Geometry check sheet. Reference: the model listing, model coordinates, mm. A direction names the side the tool comes from. Round coordinates to 2 decimals unless told otherwise and drop trailing zeros. Order: outer loops, then holes, each group sorted by start corner. A loop starts at its lowest first (then second) coordinate and runs counter-clockwise, first axis right, second up. Notation, with made-up numbers: M 75,-11.75 L 94,-11.75 A19 ccw 94,0.25 Z; hole C 60,-4.75 d1. An arc over 180 degrees is marked long. Answer as a JSON object with one key per item and string values. Group by question number.
Autodesk Fusion 360 part; units mm, degrees
sketch "Skizze1" plane through (0, 0, 0) normal (0, 0, 1) x (1, 0, 0)
  line L0 (0, 0) -> (17, 0)
  line L1 (17, 0) -> (17, 27)
  line L2 (17, 27) -> (0, 27)
  line L3 (0, 27) -> (0, 0)
  line L4 (14, 27) -> (12.5, 25.5)
  line L5 (12.5, 25.5) -> (4.5, 25.5)
  line L6 (4.5, 25.5) -> (3, 27)
  line L7 (4.5, 27) -> (12.5, 27)
  line L8 (12.5, 27) -> (12.5, 21)
  line L9 (12.5, 21) -> (4.5, 21)
  line L10 (4.5, 21) -> (4.5, 27)
  circle A0 centre (2, 25) radius 0.5
  circle A1 centre (15, 25) radius 0.5
  circle A2 centre (2, 2) radius 0.5
  circle A3 centre (15, 2) radius 0.5
  circle A4 centre (7.23, 2) radius 0.5
  circle A5 centre (9.77, 2) radius 0.5
  line L11 (8.5, 0) -> (8.5, 3.6203)
  circle A6 centre (1.5, 5.5) radius 0.5
  circle A7 centre (1.5, 8.04) radius 0.5
  circle A8 centre (1.5, 15.66) radius 0.5
  circle A9 centre (1.5, 18.2) radius 0.5
  dimension "d1" = 17
  dimension "d2" = 27
  dimension "d3" = 3
  dimension "d4" = 3
  dimension "d5" = 45
  dimension "d6" = 45
  dimension "d7" = 1.5
  dimension "d8" = 8
  dimension "d9" = 6
  dimension "d10" = 4.5
  dimension "d17" = 1
  dimension "d18" = 2
  dimension "d19" = 2
  dimension "d22" = 13
  dimension "d23" = -23
  dimension "d24" = 1
  dimension "d25" = 2
  dimension "d28" = 2.54
  dimension "d29" = 0
  dimension "d30" = 1
  dimension "d31" = 5.5
  dimension "d32" = 1.5
  dimension "d35" = 0
  dimension "d36" = 2.54
  dimension "d39" = 0
  dimension "d40" = 10.16
extrude "Extrusion2" add sketch "Skizze1" along normal blind 4 contours L2 L5 L7 L8 L10 | L5 L8 L9 L10
extrude "Extrusion3" cut sketch "Skizze1" along normal blind 1.6 contours L2 L5 L7 L8 L10
extrude "Extrusion4" add sketch "Skizze1" along normal blind 1.6 contours L0 L1 L2 L3 L4 L6 L8 L9 L10
sketch "Skizze2" plane through (0, 0, 1.6) normal (0, 0, 1) x (-1, 0, 0)
  circle A0 centre (-1.5, -15.66) radius 0.5
  circle A1 centre (-2, -2) radius 0.5
  circle A2 centre (-1.5, -8.04) radius 0.5
  circle A3 centre (-15, -25) radius 0.5
  circle A4 centre (-1.5, -18.2) radius 0.5
  circle A5 centre (-7.23, -2) radius 0.5
  circle A6 centre (-1.5, -5.5) radius 0.5
  circle A7 centre (-15, -2) radius 0.5
  circle A8 centre (-9.77, -2) radius 0.5
  circle A9 centre (-2, -25) radius 0.5
  line L0 (-4.5, -21) -> (-4.5, -25.5)
  line L1 (-4.5, -25.5) -> (-3, -27)
  line L2 (-3, -27) -> (0, -27)
  line L3 (0, -27) -> (0, 0)
  line L4 (0, 0) -> (-17, 0)
  line L5 (-17, 0) -> (-17, -27)
  line L6 (-17, -27) -> (-14, -27)
  line L7 (-14, -27) -> (-12.5, -25.5)
  line L8 (-12.5, -25.5) -> (-12.5, -21)
  line L9 (-12.5, -21) -> (-4.5, -21)
  line L10 (-4.75, -3.5) -> (-12.25, -3.5)
  line L11 (-12.25, -3.5) -> (-12.25, 7.5)
  line L12 (-12.25, 7.5) -> (-4.75, 7.5)
  line L13 (-4.75, 7.5) -> (-4.75, -3.5)
  line L14 (-4.75, 0) -> (-12.25, 0)
  line L15 (0, 0) -> (-17, 0)
  dimension "d43" = 7.5
  dimension "d44" = 11
  dimension "d45" = 3.5
extrude "Extrusion5" [suppressed]
1) Sectioned sample at D-D (x = 9.77). Record the boundary of the cut face in (y, z).
2) Sectioned sample at A-A (y = 2). Record the boundary of the cut face in (x, z).
3) Sectioned sample at B-B (y = 18.2). Record the boundary of the cut face in (x, z).
4) Sectioned sample at C-C (x = 15). Record the boundary of the cut face in (y, z), then the cut area to 3 significant figures.
5) Release check for a two-part mould opening along X. For faces 4 (the flat face through (9, 21, 3)), 5 (the cylindrical face through (1.5, 2, 0.8)), 6 (the flat face through (4.5, 24, 3)), 7 (the flat face through (12.5, 24, 3)) record: +X half, -X half, draft (parallel to the pull), parting line (faces both ways), or undercut.
6) Go/stop test with flat-tipped pins: P1, Ø1.6, axis at x = 8.5, y = 26, coming from the -Z side; P2, Ø8.5, axis at x = 12.5, y = 11, coming from the +Z side; P3, Ø1.9, axis at y = 25, z = 3, coming from the -X side; P4, Ø1.2, axis at x = 9.5, z = 3, coming from the -Y side. Record where each tip stops, or that it passes through.
7) Thickness scan on line 1 along Z through (x, y) = (16, 26.25); line 2 along Y through (x, z) = (7, 3.85); line 3 along Y through (x, z) = (5.25, 1.2). Record the ranges inside material, lowest first. Write a range as [from, to].
8) Set-up check for faces 1 (the flat face through (8, 0, 1)), 2 (the flat face through (9, 25.5, 1)), 3 (the flat face through (13, 26, 1)): record each of +Z, -Z, +X, -X, +Y, -Y from which the full face is reachable in a straight line by a thin tool's end or side.
Final values:
{
 "1": {"outline": "M 0,0 L 1.5,0 L 1.5,1.6 L 0,1.6 Z; M 2.5,0 L 25.5,0 L 25.5,1.6 L 27,1.6 L 27,4 L 21,4 L 21,1.6 L 2.5,1.6 Z"},
 "2": {"outline": "M 0,0 L 1.5,0 L 1.5,1.6 L 0,1.6 Z; M 2.5,0 L 6.73,0 L 6.73,1.6 L 2.5,1.6 Z; M 7.73,0 L 9.27,0 L 9.27,1.6 L 7.73,1.6 Z; M 10.27,0 L 14.5,0 L 14.5,1.6 L 10.27,1.6 Z; M 15.5,0 L 17,0 L 17,1.6 L 15.5,1.6 Z"},
 "3": {"outline": "M 0,0 L 1,0 L 1,1.6 L 0,1.6 Z; M 2,0 L 17,0 L 17,1.6 L 2,1.6 Z"},
 "4": {"outline": "M 0,0 L 1.5,0 L 1.5,1.6 L 0,1.6 Z; M 2.5,0 L 24.5,0 L 24.5,1.6 L 2.5,1.6 Z; M 25.5,0 L 27,0 L 27,1.6 L 25.5,1.6 Z", "area": "40.0 mm^2"},
 "5": {"face 4": "draft", "face 5": "undercut", "face 6": "-X half", "face 7": "+X half"},
 "6": {"P1": "stops at z = 0", "P2": "stops at z = 1.6", "P3": "stops at x = 4.5", "P4": "stops at y = 21"},
 "7": {"line 1": "z = [0, 1.6]", "line 2": "y = [21, 27]", "line 3": "y = [0, 25.5]"},
 "8": {"face 1": "+Z, -Z, +X, -X, -Y", "face 2": "-Z, +Y", "face 3": "+Z, -Z, +Y"}
}
